Geometry check sheet. Reference: the model listing, model coordinates, mm. Round coordinates to 2 decimals unless told otherwise and drop trailing zeros. Order: outer loops, then holes, each group sorted by start corner. A loop starts at its lowest first (then second) coordinate and runs counter-clockwise, first axis right, second up.
(1) Sectioned sample at B-B (y = 0.95). Record the boundary of the cut face in (x, z).
(2) Go/stop test with a flat-tipped pin: pin 1 (2 mm diameter, centred on x = -41, y = 1, fed in from +Z). Record where the tip stops, or that it passes through.
(3) Sectioned sample at A-A (x = 30). Record the boundary of the cut face in (y, z).
(4) Release check for a two-part mould opening along X. For faces 1 (the face through (-1, 4, -4.9)), 2 (the face through (1.796, 4.507, -0.713)), 3 (the face through (51.4, 4, 0)) record: +X half, -X half, draft (parallel to the pull), parting line (faces both ways), or undercut.
(5) Material ranges on line 1 along Y through (x, z) = (43, -3.5); line 2 along X through (y, z) = (2.7, 1.75); line 3 along Z through (x, y) = (20.5, 2.8), recorded low to high.
from build123d import *

# Parameters (mm, degrees)
SKETCH1_W           = 98.8
SKETCH1_H           = 5.8
BOSS_EXTRUDE1_DEPTH = 3
SKETCH2_W           = 100.8
SKETCH2_H           = 7.8
BOSS_EXTRUDE3_DEPTH = 2
DRAFT1_ANGLE        = 3
SKETCH3_W           = 102.8
SKETCH3_H           = 9.8
BOSS_EXTRUDE4_DEPTH = 2
FILLET1_R           = 0.5
CUT_EXTRUDE1_DEPTH  = 1


with BuildPart() as part:
    # Sketch1 → Boss-Extrude1 (new body)
    with BuildSketch(Plane(origin=(0, 0, 0), x_dir=(1, 0, 0), z_dir=(0, 1, 0))):
        Rectangle(SKETCH1_W, SKETCH1_H)
    extrude(amount=BOSS_EXTRUDE1_DEPTH)

    # Draft1
    draft1_faces = [part.faces().sort_by_distance(p)[0] for p in [
        (49.4, 1.5, 0),
        (0, 1.5, 2.9),
        (-49.4, 1.5, 0),
        (0, 1.5, -2.9),
    ]]
    draft(draft1_faces, Plane(origin=(0, 3, 0), x_dir=(0, 0, -1), z_dir=(0, -1, 0)), DRAFT1_ANGLE)



with BuildPart() as body_2:
    # Sketch2 → Boss-Extrude3 (new body)
    with BuildSketch(Plane(origin=(0, 3, 0), x_dir=(1, 0, 0), z_dir=(0, 1, 0))):
        Rectangle(SKETCH2_W, SKETCH2_H)
    extrude(amount=BOSS_EXTRUDE3_DEPTH)


with BuildPart() as part_1:
    add(part.part)

    add(body_2.part)  # Boss-Extrude4 merges body 2
    # Sketch3 → Boss-Extrude4 (add)
    with BuildSketch(Plane(origin=(0, 5, 0), x_dir=(1, 0, 0), z_dir=(0, 1, 0))):
        Rectangle(SKETCH3_W, SKETCH3_H)
    extrude(amount=-BOSS_EXTRUDE4_DEPTH)

    # Fillet1
    fillet1_edges = [part_1.edges().sort_by_distance(p)[0] for p in [
        (-51.4, 4, 4.9),
        (-51.4, 4, -4.9),
        (51.4, 4, -4.9),
        (51.4, 4, 4.9),
    ]]
    fillet(fillet1_edges, radius=FILLET1_R)

    # Sketch4 → Cut-Extrude1 (cut)
    # profile 1 of 2: a face of its own
    with BuildSketch(Plane(origin=(0, 5, 0), x_dir=(1, 0, 0), z_dir=(0, 1, 0))):
        Polygon((-2.466339169, 2.034069186), (-2.129800707, 2.034069186), (-0.96313404, -0.724143955), (0.203532626, 2.034069186), (0.540071088, 2.034069186), (-0.940698143, -1.465930814), (-0.985569938, -1.465930814), align=None)
    # profile 2 of 2: a face of its own
    with BuildSketch(Plane(origin=(0, 5, 0), x_dir=(1, 0, 0), z_dir=(0, 1, 0))):
        Polygon((2.764730543, 2.123812775), (2.828532626, 2.123812775), (2.828532626, -0.299264148), (3.23237878, -0.299264148), (3.23237878, -0.658238507), (2.828532626, -0.658238507), (2.828532626, -1.465930814), (2.514430062, -1.465930814), (2.514430062, -0.658238507), (0.854173652, -0.658238507), align=None)
        Polygon((2.514430062, -0.299264148), (2.514430062, 1.220767903), (1.471160831, -0.299264148), align=None, mode=Mode.SUBTRACT)
    extrude(amount=-CUT_EXTRUDE1_DEPTH, mode=Mode.SUBTRACT)


solid = part_1.part
Answer below:
1. outline: (-49.29, -2.79) - (49.29, -2.79) - (49.29, 2.79) - (-49.29, 2.79) - close
2. pin 1: stops at z = 2.85
3. outline: (0, -2.74) - (3, -2.9) - (3, -4.9) - (5, -4.9) - (5, 4.9) - (3, 4.9) - (3, 2.9) - (0, 2.74) - close
4. face 1: draft
4. face 2: undercut
4. face 3: +X half
5. line 1: y = 3 to 5
5. line 2: x = -49.38 to 49.38
5. line 3: z = -2.89 to 2.89
